from build123d import *

# Parameters (mm, degrees)
SKETCH1_W           = 300
SKETCH1_H           = 150
BOSS_EXTRUDE1_DEPTH = 3
CUT_EXTRUDE1_DEPTH  = 3


with BuildPart() as part:
    # Sketch1 → Boss-Extrude1 (new body)
    with BuildSketch(Plane(origin=(0, 0, 0), x_dir=(1, 0, 0), z_dir=(0, 1, 0))):
        Rectangle(SKETCH1_W, SKETCH1_H)
    extrude(amount=BOSS_EXTRUDE1_DEPTH)

    # Sketch2 → Cut-Extrude1 (cut)
    with BuildSketch(Plane(origin=(0, 3, 0), x_dir=(1, 0, 0), z_dir=(0, 1, 0))):
        with BuildLine():
            Line((-135, 67), (-15, 67))
            ThreePointArc((-15, 67), (-13, 65), (-15, 63))
            Line((-15, 63), (-135, 63))
            ThreePointArc((-135, 63), (-137, 65), (-135, 67))
        make_face()
        with BuildLine():
            Line((15, 67), (135, 67))
            ThreePointArc((135, 67), (137, 65), (135, 63))
            Line((135, 63), (15, 63))
            ThreePointArc((15, 63), (13, 65), (15, 67))
        make_face()
        with BuildLine():
            Line((15, 57), (135, 57))
            ThreePointArc((135, 57), (137, 55), (135, 53))
            Line((135, 53), (15, 53))
            ThreePointArc((15, 53), (13, 55), (15, 57))
        make_face()
        with BuildLine():
            Line((15, 47), (135, 47))
            ThreePointArc((135, 47), (137, 45), (135, 43))
            Line((135, 43), (15, 43))
            ThreePointArc((15, 43), (13, 45), (15, 47))
        make_face()
        with BuildLine():
            Line((15, 37), (135, 37))
            ThreePointArc((135, 37), (137, 35), (135, 33))
            Line((135, 33), (15, 33))
            ThreePointArc((15, 33), (13, 35), (15, 37))
        make_face()
        with BuildLine():
            Line((15, 27), (135, 27))
            ThreePointArc((135, 27), (137, 25), (135, 23))
            Line((135, 23), (15, 23))
            ThreePointArc((15, 23), (13, 25), (15, 27))
        make_face()
        with BuildLine():
            Line((15, 17), (135, 17))
            ThreePointArc((135, 17), (137, 15), (135, 13))
            Line((135, 13), (15, 13))
            ThreePointArc((15, 13), (13, 15), (15, 17))
        make_face()
        with BuildLine():
            Line((15, 7), (135, 7))
            ThreePointArc((135, 7), (137, 5), (135, 3))
            Line((135, 3), (15, 3))
            ThreePointArc((15, 3), (13, 5), (15, 7))
        make_face()
        with BuildLine():
            Line((15, -3), (135, -3))
            ThreePointArc((135, -3), (137, -5), (135, -7))
            Line((135, -7), (15, -7))
            ThreePointArc((15, -7), (13, -5), (15, -3))
        make_face()
        with BuildLine():
            Line((15, -13), (135, -13))
            ThreePointArc((135, -13), (137, -15), (135, -17))
            Line((135, -17), (15, -17))
            ThreePointArc((15, -17), (13, -15), (15, -13))
        make_face()
        with BuildLine():
            Line((15, -23), (135, -23))
            ThreePointArc((135, -23), (137, -25), (135, -27))
            Line((135, -27), (15, -27))
            ThreePointArc((15, -27), (13, -25), (15, -23))
        make_face()
        with BuildLine():
            Line((15, -33), (135, -33))
            ThreePointArc((135, -33), (137, -35), (135, -37))
            Line((135, -37), (15, -37))
            ThreePointArc((15, -37), (13, -35), (15, -33))
        make_face()
        with BuildLine():
            Line((15, -43), (135, -43))
            ThreePointArc((135, -43), (137, -45), (135, -47))
            Line((135, -47), (15, -47))
            ThreePointArc((15, -47), (13, -45), (15, -43))
        make_face()
        with BuildLine():
            Line((15, -53), (135, -53))
            ThreePointArc((135, -53), (137, -55), (135, -57))
            Line((135, -57), (15, -57))
            ThreePointArc((15, -57), (13, -55), (15, -53))
        make_face()
        with BuildLine():
            Line((15, -63), (135, -63))
            ThreePointArc((135, -63), (137, -65), (135, -67))
            Line((135, -67), (15, -67))
            ThreePointArc((15, -67), (13, -65), (15, -63))
        make_face()
        with BuildLine():
            Line((-135, 57), (-15, 57))
            ThreePointArc((-15, 57), (-13, 55), (-15, 53))
            Line((-15, 53), (-135, 53))
            ThreePointArc((-135, 53), (-137, 55), (-135, 57))
        make_face()
        with BuildLine():
            Line((-135, 47), (-15, 47))
            ThreePointArc((-15, 47), (-13, 45), (-15, 43))
            Line((-15, 43), (-135, 43))
            ThreePointArc((-135, 43), (-137, 45), (-135, 47))
        make_face()
        with BuildLine():
            Line((-135, 37), (-15, 37))
            ThreePointArc((-15, 37), (-13, 35), (-15, 33))
            Line((-15, 33), (-135, 33))
            ThreePointArc((-135, 33), (-137, 35), (-135, 37))
        make_face()
        with BuildLine():
            Line((-135, 27), (-15, 27))
            ThreePointArc((-15, 27), (-13, 25), (-15, 23))
            Line((-15, 23), (-135, 23))
            ThreePointArc((-135, 23), (-137, 25), (-135, 27))
        make_face()
        with BuildLine():
            Line((-135, 17), (-15, 17))
            ThreePointArc((-15, 17), (-13, 15), (-15, 13))
            Line((-15, 13), (-135, 13))
            ThreePointArc((-135, 13), (-137, 15), (-135, 17))
        make_face()
        with BuildLine():
            Line((-135, 7), (-15, 7))
            ThreePointArc((-15, 7), (-13, 5), (-15, 3))
            Line((-15, 3), (-135, 3))
            ThreePointArc((-135, 3), (-137, 5), (-135, 7))
        make_face()
        with BuildLine():
            Line((-135, -3), (-15, -3))
            ThreePointArc((-15, -3), (-13, -5), (-15, -7))
            Line((-15, -7), (-135, -7))
            ThreePointArc((-135, -7), (-137, -5), (-135, -3))
        make_face()
        with BuildLine():
            Line((-135, -13), (-15, -13))
            ThreePointArc((-15, -13), (-13, -15), (-15, -17))
            Line((-15, -17), (-135, -17))
            ThreePointArc((-135, -17), (-137, -15), (-135, -13))
        make_face()
        with BuildLine():
            Line((-135, -23), (-15, -23))
            ThreePointArc((-15, -23), (-13, -25), (-15, -27))
            Line((-15, -27), (-135, -27))
            ThreePointArc((-135, -27), (-137, -25), (-135, -23))
        make_face()
        with BuildLine():
            Line((-135, -33), (-15, -33))
            ThreePointArc((-15, -33), (-13, -35), (-15, -37))
            Line((-15, -37), (-135, -37))
            ThreePointArc((-135, -37), (-137, -35), (-135, -33))
        make_face()
        with BuildLine():
            Line((-135, -43), (-15, -43))
            ThreePointArc((-15, -43), (-13, -45), (-15, -47))
            Line((-15, -47), (-135, -47))
            ThreePointArc((-135, -47), (-137, -45), (-135, -43))
        make_face()
        with BuildLine():
            Line((-135, -53), (-15, -53))
            ThreePointArc((-15, -53), (-13, -55), (-15, -57))
            Line((-15, -57), (-135, -57))
            ThreePointArc((-135, -57), (-137, -55), (-135, -53))
        make_face()
        with BuildLine():
            Line((-135, -63), (-15, -63))
            ThreePointArc((-15, -63), (-13, -65), (-15, -67))
            Line((-15, -67), (-135, -67))
            ThreePointArc((-135, -67), (-137, -65), (-135, -63))
        make_face()
        with BuildLine():
            Line((-7.5, -59.5), (-7.5, 59.5))
            ThreePointArc((-7.5, 59.5), (0, 67), (7.5, 59.5))
            Line((7.5, 59.5), (7.5, -59.5))
            ThreePointArc((7.5, -59.5), (0, -67), (-7.5, -59.5))
        make_face()
    extrude(amount=-CUT_EXTRUDE1_DEPTH, mode=Mode.SUBTRACT)


solid = part.part
Input: part model. Units: mm. Frame: model coordinates. A direction names the side the tool comes from. Give positions to 0.01 mm unless a question says otherwise; leave off trailing zeros. Use one line per item in the form item = value.
1) Reachability of faces 3 (the flat face through (31, 3, -18)), 4 (the cylindrical face through (0, 2, -67)) from +Z, -Z, +X, -X, +Y, -Y: full face, straight path, thin tool, end or side. Return the list, or none.
Response values:
face_3 = +Z, -Z, +X, -X, +Y
face_4 = +Y, -Y
2) Section A-A, the plane x = -101. Count the separate pieces of the cut face and the enclosed holes in it, and give its area (3 significant figures).
Response values:
separate_pieces = 15
enclosed_holes = 0
area = 282 mm^2
3) First-contact query: pin 1 Ø10 at (x, z) = (57.5, -13) entering from -Y. Flat tip, straight axial feed; report the tip coordinate or a pass-through.
Response values:
pin_1 = 0
4) Line query: probe 1 along X at (y, z) = (1.8, -45); probe 2 along X at (y, z) = (2.85, -12); probe 3 along X at (y, z) = (1.85, -26). Output: solid intervals per line, ascending.
Response values:
probe_1 = -150 to -137, -13 to -7.5, 7.5 to 13, 137 to 150
probe_2 = -150 to -7.5, 7.5 to 150
probe_3 = -150 to -136.73, -13.27 to -7.5, 7.5 to 13.27, 136.73 to 150
5) Mould query, pull axis X, two halves, no side actions, for faces 1 (the cylindrical face through (0, 2, 67)), 2 (the flat face through (31, 0, -18)). Classes: pulls with the +X half, pulls with the -X half, needs draft (parallel to the pull), parting line crosses it, or undercut.
Response values:
face_1 = undercut
face_2 = needs draft
